Here's how the part is built. I have some questions about the finished solid (model axes, mm). Face numbers are marked on the shaded views. A direction names the side the tool comes from. Round coordinates to 2 decimals unless told otherwise and drop trailing zeros. Loops run counter-clockwise (first coordinate to the right, second up) from the corner with the lowest first, then second, coordinate; pieces in that order, holes last. Notation, with made-up numbers: (83, 1.5) - (141, 1.5) arc R11 ccw to (141, 13.5) - close; hole circle Ø8 at (-24, 13). An arc over 180 degrees is marked (long way). Answer as a JSON object with one key per item and string values. Group by question number.
1) If we mould it in two halves opening along X, with no side actions, what happens to the marked faces 1, 2 and 3? For each: pulls with the +X half, pulls with the -X half, needs draft (parallel to the pull), parting line crosses it, or undercut.
2) If I drill on line 1 along Z through (x, y) = (1.6, 13); line 2 along X through (y, z) = (6, 9); line 3 along Y through (x, z) = (6, 2.05), over which ranges is the centre line in solid material (lowest first)? Write a range as [from, to].
3) I want a section at C-C, the plane y = 5.25. Please give me the cut outline in (x, z).
4) Which directions (+Z, -Z, +X, -X, +Y, -Y) give clear straight access to the entire face, cutting with the end or side of a thin tool? Please do the marked faces 4, 5 and 6.
5) I want a section at A-A, the plane x = 15. Please give me the cut outline in (y, z).
6) I want a section at B-B, the plane z = 10.75. Please give me the cut outline in (x, y), then the cut area to 3 significant figures.
7) I want a section at D-D, the plane z = 6. Please give me the cut outline in (x, y), then the cut area to 3 significant figures.
8) Will these pins go through, and if not, where does the flat tip stop? P1, Ø1.7, axis at y = 14.5, z = 6.5, coming from the +X side; P2, Ø6, axis at x = 14.5, z = 5, coming from the -Y side; P3, Ø2, axis at x = 22, z = 7.5, coming from the -Y side; P4, Ø3, axis at x = 16.5, y = 10.5, coming from the +Z side.
from build123d import *

# Parameters (mm, degrees)
F0_W      = 21
F0_H      = 18
F1_DEPTH  = 3
F2_W      = 2.85
F2_H      = 18
F3_DEPTH  = 9
F4_R      = 6
F5_R      = 1.75
F6_DEPTH  = 21.001
F7_R      = 5
F8_R      = 1.75
F9_DEPTH  = 3.001
F10_DEPTH = 2
F12_DEPTH = 2.5


with BuildPart() as f1:
    # F0 (on Top) → F1 (new body)
    with BuildSketch(Plane.XY):
        with Locations((10.5, 9)):
            Rectangle(F0_W, F0_H)
    extrude(amount=F1_DEPTH)

    # F2 (on face) → F3 (join)
    with BuildSketch(Plane.XY.offset(3)):
        with Locations((1.425, 9)):
            Rectangle(F2_W, F2_H)
        with Locations((19.575, 9)):
            Rectangle(F2_W, F2_H)
    extrude(amount=F3_DEPTH)

    # F4
    f4_edges = [f1.edges().sort_by_distance(p)[0] for p in [
        (0, 0, 6),
    ]]
    fillet(f4_edges, radius=F4_R)

    # F5 (on face) → F6 (cut, through all)
    with BuildSketch(Plane(origin=(0, 0, 0), x_dir=(0, -1, 0), z_dir=(-1, 0, 0))):
        with Locations((-13, 7)):
            Circle(F5_R)
        Polygon((0, 12), (-8, 12), (0, 3), align=None)
    extrude(amount=-F6_DEPTH, mode=Mode.SUBTRACT)

    # F7
    f7_edges = [f1.edges().sort_by_distance(p)[0] for p in [
        (1.425, 18, 12),
        (19.575, 18, 12),
        (1.425, 8, 12),
        (19.575, 8, 12),
    ]]
    fillet(f7_edges, radius=F7_R)

    # F8 (on face) → F9 (cut, through all)
    with BuildSketch(Plane.XY.offset(3)):
        with Locations((6, 6)):
            Circle(F8_R)
        with Locations((15, 6)):
            Circle(F8_R)
    extrude(amount=-F9_DEPTH, mode=Mode.SUBTRACT)

    # F10 (add): a face of the model
    f10_faces = [f1.faces().sort_by_distance(p)[0] for p in [
        (21, 9.8993100801, 5.1016484072),
    ]]
    extrude(f10_faces, amount=F10_DEPTH)

    # F11 (on face) → F12 (cut)
    with BuildSketch(Plane.YZ.offset(23)):
        Polygon((15.85, 5.3545517328), (15.85, 8.6454482672), (13, 10.2908965344), (10.15, 8.6454482672), (10.15, 5.3545517328), (13, 3.7091034656), align=None)
    extrude(amount=-F12_DEPTH, mode=Mode.SUBTRACT)


solid = f1.part
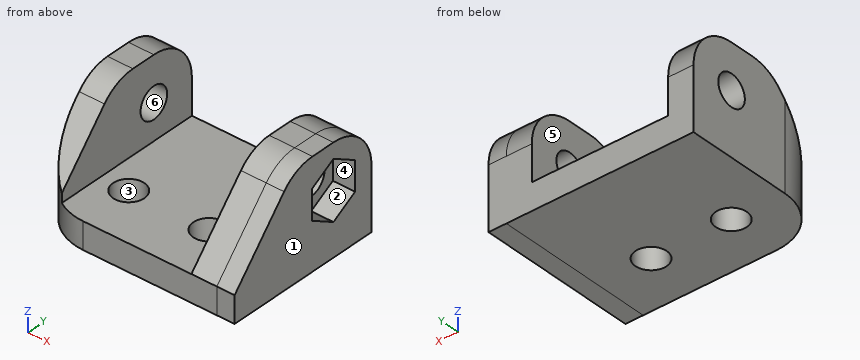
Outcome:
{
 "1": {"face 1": "pulls with the +X half", "face 2": "needs draft", "face 3": "undercut"},
 "2": {"line 1": "[0, 5.25], [8.75, 12]", "line 2": "[0, 2.85], [18.15, 23]", "line 3": "[0, 4.25], [7.75, 18]"},
 "3": {"outline": "(0.05, 0) - (4.42, 0) - (4.42, 3) - (2.85, 3) - (2.85, 8.91) - (0.05, 8.91) - close; (7.58, 0) - (13.42, 0) - (13.42, 3) - (7.58, 3) - close; (16.58, 0) - (23, 0) - (23, 8.91) - (18.15, 8.91) - (18.15, 3) - (16.58, 3) - close"},
 "4": {"face 4": "+X", "face 5": "+Z, +Y, -Y", "face 6": "+X, -X"},
 "5": {"outline": "(0, 0) - (4.25, 0) - (4.25, 3) - (0, 3) - close; (7.75, 0) - (18, 0) - (18, 3) - (7.75, 3) - close"},
 "6": {"outline": "(0, 6.94) - (2.85, 6.94) - (2.85, 16.31) - (0, 16.31) - close; (18.15, 6.94) - (23, 6.94) - (23, 16.31) - (18.15, 16.31) - close", "area": "72.1 mm^2"},
 "7": {"outline": "(0, 6) arc R6 ccw to (1.01, 2.67) - (2.85, 2.67) - (2.85, 11.56) - (0, 11.56) - close; (0, 14.44) - (2.85, 14.44) - (2.85, 18) - (0, 18) - close; (18.15, 2.67) - (23, 2.67) - (23, 10.15) - (20.5, 10.15) - (20.5, 11.56) - (18.15, 11.56) - close; (18.15, 14.44) - (20.5, 14.44) - (20.5, 15.85) - (23, 15.85) - (23, 18) - (18.15, 18) - close", "area": "87.8 mm^2"},
 "8": {"P1": "x = 20.5", "P2": "y = 0", "P3": "y = 3.11", "P4": "z = 3"}
}
